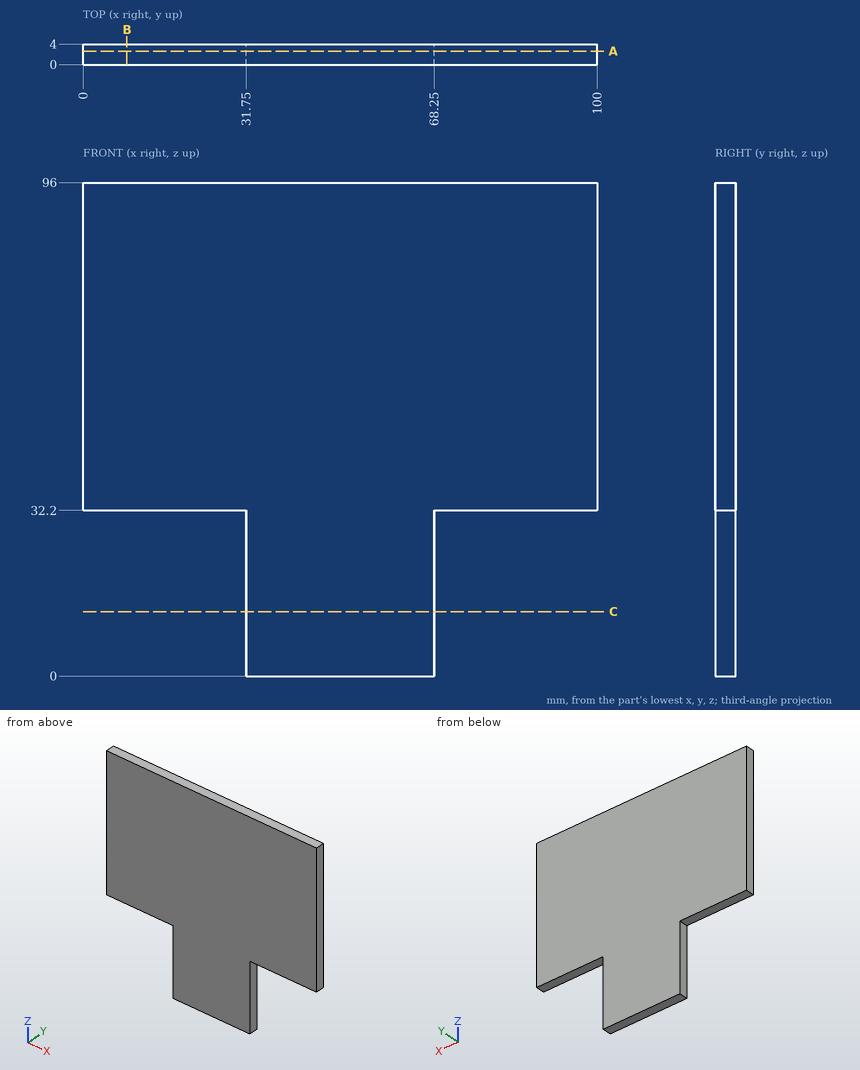
For this review, use the dimensioned drawing (mm, ordinates from the lowest corner) and the shaded views. Round coordinates to 2 decimals unless told otherwise and drop trailing zeros. Write each loop counter-clockwise with the first axis right and the second up, starting at its lowest first coordinate (ties: lowest second). Pieces come first, ordered by that corner, then holes. Notation, with made-up numbers: M 36,70 L 51,70 A6 ccw 51,76 Z; hole C 26,-11.5 d5. An arc over 180 degrees is marked long. Write item = value, one per line. Start each with the question number.
(1) Clearance check with flat-ended pins moving along their axes: pin 1 Ø2 at (y, z) = (1.5, 20) entering from +X; pin 2 Ø2 at (y, z) = (0.5, 23.5) entering from -X; pin 3 Ø1.2 at (x, y) = (79.5, 1.5) entering from -Z. State where each tip first meets the part, or that it passes through.
(2) We need section A-A (y = 2.6). Give the boundary of the cut face in (x, z), then the cut area to 3 significant figures.
(3) We need section B-B (x = 8.5). Give the boundary of the cut face in (y, z), then the cut area to 3 significant figures.
(4) We need section C-C (z = 12.5). Give the boundary of the cut face in (x, y), then the cut area to 3 significant figures.
(5) For line 1 along X through (y, z) = (0.5, 21); line 2 along Z through (x, y) = (71, 2.15), list the stretches that pass through material, from the lowest coordinate up.
Results found:
q1.pin_1 = 68.25
q1.pin_2 = 31.75
q1.pin_3 = 32.2
q2.outline = M 0,32.2 L 31.75,32.2 L 31.75,0 L 68.25,0 L 68.25,32.2 L 100,32.2 L 100,96 L 0,96 Z
q2.area = 7,560 mm²
q3.outline = M 0,32.2 L 4,32.2 L 4,96 L 0,96 Z
q3.area = 255 mm²
q4.outline = M 31.75,0 L 68.25,0 L 68.25,4 L 31.75,4 Z
q4.area = 146 mm²
q5.line_1 = 31.75 to 68.25
q5.line_2 = 32.2 to 96
